```python
from build123d import *

# Parameters (mm, degrees)
SKETCH1_W           = 6
SKETCH1_H           = 3.5
BOSS_EXTRUDE1_DEPTH = 3.5
SKETCH2_W           = 3
SKETCH2_H           = 1.5
BOSS_EXTRUDE2_DEPTH = 0.7
SKETCH3_W           = 0.3
SKETCH3_H           = 1.5
BOSS_EXTRUDE3_DEPTH = 1
SKETCH4_W           = 0.3
SKETCH4_H           = 1.5
BOSS_EXTRUDE4_DEPTH = 0.6


with BuildPart() as part:
    # Sketch1 → Boss-Extrude1 (new body)
    with BuildSketch(Plane.XY):
        Rectangle(SKETCH1_W, SKETCH1_H)
    extrude(amount=BOSS_EXTRUDE1_DEPTH)

    # Sketch2 → Boss-Extrude2 (add)
    with BuildSketch(Plane.XY.offset(3.5)):
        Rectangle(SKETCH2_W, SKETCH2_H)
    extrude(amount=BOSS_EXTRUDE2_DEPTH)

    # Sketch3 → Boss-Extrude3 (add)
    with BuildSketch(Plane.ZY.offset(3)):
        with Locations((0.15, 0)):
            Rectangle(SKETCH3_W, SKETCH3_H)
    boss_extrude3 = extrude(amount=BOSS_EXTRUDE3_DEPTH)

    # Sketch4 → Boss-Extrude4 (add)
    with BuildSketch(Plane.XY.offset(0.3)):
        with Locations((-3.15, 0)):
            Rectangle(SKETCH4_W, SKETCH4_H)
    boss_extrude4 = extrude(amount=BOSS_EXTRUDE4_DEPTH)

    # Mirror1: Boss-Extrude3, Boss-Extrude4 across plane
    add(boss_extrude3.mirror(Plane(origin=(0, 0, 0), x_dir=(0, 0, 1), z_dir=(1, 0, 0))))
    add(boss_extrude4.mirror(Plane(origin=(0, 0, 0), x_dir=(0, 0, 1), z_dir=(1, 0, 0))))


solid = part.part
```
CAD build for the part. Positions are in the model's coordinates, mm. Coordinates: 2 decimals unless noted, no trailing zeros. Order: outer loops, then holes, each group sorted by start corner. A loop starts at its lowest first (then second) coordinate and runs counter-clockwise, first axis right, second up. Notation, with made-up numbers: (58.25, 1) - (94.25, 1) arc R12 cw to (94.25, 5) - close; hole circle Ø5 at (27.5, 38.25). An arc over 180 degrees is marked (long way). Answer in a Markdown table with one row per item.
1. Slice it at C-C, the plane x = 0.75. List the corners of the cut face in (y, z).
Answer:
| item | result |
|---|---|
| outline | (-1.75, 0) - (1.75, 0) - (1.75, 3.5) - (0.75, 3.5) - (0.75, 4.2) - (-0.75, 4.2) - (-0.75, 3.5) - (-1.75, 3.5) - close |
2. Slice it at A-A, the plane y = -0.25. List the corners of the cut face in (x, z), then the cut area to 3 significant figures.
Answer:
| item | result |
|---|---|
| outline | (-4, 0) - (4, 0) - (4, 0.3) - (3.3, 0.3) - (3.3, 0.9) - (3, 0.9) - (3, 3.5) - (1.5, 3.5) - (1.5, 4.2) - (-1.5, 4.2) - (-1.5, 3.5) - (-3, 3.5) - (-3, 0.9) - (-3.3, 0.9) - (-3.3, 0.3) - (-4, 0.3) - close |
| area | 24.1 mm² |
3. Slice it at D-D, the plane z = 3.35. List the corners of the cut face in (x, y).
Answer:
| item | result |
|---|---|
| outline | (-3, -1.75) - (3, -1.75) - (3, 1.75) - (-3, 1.75) - close |
4. Flat gauge pins, fed straight in: P1, Ø0.8, axis at y = 0, z = 3.5, coming from the -X side; P2, Ø0.6, axis at x = 0, z = 4, coming from the -Y side; P3, Ø0.6, axis at y = 0, z = 4, coming from the +X side. Where does each tip first touch, or does it go through?
Answer:
| item | result |
|---|---|
| P1 | x = -3 |
| P2 | y = -0.75 |
| P3 | x = 1.5 |
5. Drill centre lines: L1, parallel to Z at x = -2, y = -1.1; L2, parallel to X at y = -1, z = 2.9; L3, parallel to Z at x = 3.25, y = -0.55. Where is each one in solid material? Low to high. Write a range as from..to.
Answer:
| item | result |
|---|---|
| L1 | 0..3.5 |
| L2 | -3..3 |
| L3 | 0..0.9 |
6. Slice it at B-B, the plane z = 0.4. List the corners of the cut face in (x, y).
Answer:
| item | result |
|---|---|
| outline | (-3.3, -0.75) - (-3, -0.75) - (-3, -1.75) - (3, -1.75) - (3, -0.75) - (3.3, -0.75) - (3.3, 0.75) - (3, 0.75) - (3, 1.75) - (-3, 1.75) - (-3, 0.75) - (-3.3, 0.75) - close |
